Check sheet for the modelled part. Datum: model origin and axes. Units: mm. A direction names the side the tool comes from. Give positions to 0.01 mm unless a question says otherwise; leave off trailing zeros. Order: outer loops, then holes, each group sorted by start corner. A loop starts at its lowest first (then second) coordinate and runs counter-clockwise, first axis right, second up.
```python
from build123d import *

# Parameters (mm, degrees)
F1_DEPTH = 12.5
F2_W     = 2
F2_H     = 19.5
F3_DEPTH = 16.5
F4_SIZE  = 2
F5_R     = 3
F6_DEPTH = 21.001


with BuildPart() as f1:
    # F0 (on Top) → F1 (new body, symmetric)
    with BuildSketch(Plane.XY):
        with BuildLine():
            Line((49.5, 2.330127), (33.928203, 11.320508))
            ThreePointArc((33.928203, 11.320508), (29.104584, 13.318517), (23.928203, 14))
            Line((23.928203, 14), (-17, 14))
            ThreePointArc((-17, 14), (-22.575922, 5.784353), (-12.881908, 3.636364))
            ThreePointArc((-12.881908, 3.636364), (-11.296538, 4.646602), (-9.450166, 5))
            Line((-9.450166, 5), (0, 5))
            ThreePointArc((0, 5), (3.535534, 3.535534), (5, 0))
            Line((5, 0), (5, -2))
            ThreePointArc((5, -2), (6.464466, -5.535534), (10, -7))
            Line((10, -7), (47, -7))
            ThreePointArc((47, -7), (51.829629, -3.294095), (49.5, 2.330127))
        make_face()
    extrude(amount=F1_DEPTH, both=True)

    # F2 (on face) → F3 (cut)
    with BuildSketch(Plane(origin=(5, 0, 0), x_dir=(0, -1, 0), z_dir=(-1, 0, 0))):
        with Locations((1.5, 0)):
            Rectangle(F2_W, F2_H)
    extrude(amount=-F3_DEPTH, mode=Mode.SUBTRACT)

    # F4
    f4_edges = [f1.edges().sort_by_distance(p)[0] for p in [
        (41.714102, 6.825318, 12.5),
        (29.104584, 13.318517, 12.5),
        (3.464102, 14, 12.5),
        (-22.575922, 5.784353, 12.5),
        (-11.296538, 4.646602, 12.5),
        (-4.725083, 5, 12.5),
        (3.535534, 3.535534, 12.5),
        (5, -1, 12.5),
        (6.464466, -5.535534, 12.5),
        (28.5, -7, 12.5),
        (51.829629, -3.294095, 12.5),
        (41.714102, 6.825318, -12.5),
        (29.104584, 13.318517, -12.5),
        (3.464102, 14, -12.5),
        (-22.575922, 5.784353, -12.5),
        (-11.296538, 4.646602, -12.5),
        (-4.725083, 5, -12.5),
        (3.535534, 3.535534, -12.5),
        (5, -1, -12.5),
        (6.464466, -5.535534, -12.5),
        (28.5, -7, -12.5),
        (51.829629, -3.294095, -12.5),
    ]]
    chamfer(f4_edges, length=F4_SIZE)

    # F5 (on face) → F6 (cut, through all)
    with BuildSketch(Plane.XZ.offset(7)):
        with Locations((44, 0)):
            Circle(F5_R)
    extrude(amount=-F6_DEPTH, mode=Mode.SUBTRACT)


solid = f1.part
```
(1) Sectioned sample at D-D (y = 8). Enter the section's corners in (x, z).
(2) Release check for a two-part mould opening along Y. For faces 4 (the face through (14, 4, 12.5)), 5 (the face through (13, -2.5, 0)), 6 (the face through (7.31, -4.63, -11.74)) record: released by +Y, released by -Y, zero draft, split by the parting line, or undercut.
(3) Go/stop test with flat-tipped pins: P1, Ø8, axis at x = 44, z = 0, coming from the +Y side; P2, Ø3, axis at x = -4, z = 3, coming from the -Y side; P3, Ø5, axis at y = 11, z = -6.5, coming from the -X side. Record where each tip stops, or that it passes through.
(4) Sectioned sample at A-A (z = 1). Enter the section's corners in (x, y).
(5) Sectioned sample at B-B (x = 44). Enter the section's corners in (y, z).
(6) Sectioned sample at C-C (z = -4.5). Enter the section's corners in (x, y), plus the area to 3 significant figures.
(7) Thickness scan on L1, parallel to Y at x = 11, z = -5.5; L2, parallel to Z at x = 44, y = -1.75; L3, parallel to X at y = 3, z = 0. Record the ranges inside material, lowest first.
(8) Tool access check on faces 1 (the face through (3, 4, 0)), 2 (the face through (13, -1, 9.75)), 3 (the face through (5, -0.3, 0)). Record the directions out of +Z, -Z, +X, -X, +Y, -Y that give a thin tool (end or side, any length) a straight path to the whole face; none if there is none.
Values follow:
1. outline: (-23, -10.5) - (-21, -12.5) - (35.68, -12.5) - (39.68, -10.5) - (39.68, 10.5) - (35.68, 12.5) - (-21, 12.5) - (-23, 10.5) - close
2. face 4: zero draft
2. face 5: undercut
2. face 6: released by -Y
3. P1: stops at y = 7.81
3. P2: stops at y = 5
3. P3: stops at x = -22.98
4. outline: (-17, 14) arc R6 ccw (long way) to (-12.88, 3.64) arc R5 cw to (-9.45, 5) - (0, 5) arc R5 cw to (5, 0) - (5, -0.5) - (21.5, -0.5) - (21.5, -2.5) - (5.03, -2.5) arc R5 ccw to (10, -7) - (41.17, -7) - (41.17, 7.14) - (33.93, 11.32) arc R20 ccw to (23.93, 14) - close; (46.83, -7) - (47, -7) arc R5 ccw to (49.5, 2.33) - (46.83, 3.87) - close
5. outline: (-7, -10.5) - (-5, -12.5) - (3.2, -12.5) - (5.51, -10.5) - (5.51, -3) - (-7, -3) - close; (-7, 3) - (5.51, 3) - (5.51, 10.5) - (3.2, 12.5) - (-5, 12.5) - (-7, 10.5) - close
6. outline: (-17, 14) arc R6 ccw (long way) to (-12.88, 3.64) arc R5 cw to (-9.45, 5) - (0, 5) arc R5 cw to (5, 0) - (5, -0.5) - (21.5, -0.5) - (21.5, -2.5) - (5.03, -2.5) arc R5 ccw to (10, -7) - (47, -7) arc R5 ccw to (49.5, 2.33) - (33.93, 11.32) arc R20 ccw to (23.93, 14) - close
6. area: 1,060 mm2
7. L1: y = -7 to -2.5, -0.5 to 14
7. L2: z = -12.5 to -3, 3 to 12.5
7. L3: x = -20.32 to -13.68, 4 to 41, 47 to 48.34
8. face 1: +Z, -Z, -Y
8. face 2: -X
8. face 3: +Z, -Z, -X, -Y
